from build123d import *

# Parameters (mm, degrees)
BOSS_EXTRUDE2_DEPTH   = 80
SKETCH3_W             = 20
SKETCH3_H             = 50
BOSS_EXTRUDE3_DEPTH   = 50
FILLET3_R             = 25
SKETCH8_R             = 12.5
CUT_EXTRUDE1_DEPTH    = 50
SKETCH9_R             = 7.5
CUT_EXTRUDE3_DEPTH    = 50
FILLET4_R             = 2
FILLET5_R             = 2
FILLET3_OF_MIRROR14_R = 25
FILLET4_OF_MIRROR14_R = 2
FILLET5_OF_MIRROR14_R = 2


with BuildPart() as part:
    # Sketch1 → Boss-Extrude2 (new body)
    with BuildSketch(Plane(origin=(0, 0, 0), x_dir=(0, 0, -1), z_dir=(1, 0, 0))):
        Polygon((0, 0), (-80, 0), (-80, -30), (-56.339745962, -30), (-65, -15), (-15, -15), (-23.660254038, -30), (0, -30), align=None)
    boss_extrude2 = extrude(amount=BOSS_EXTRUDE2_DEPTH)

    # Sketch3 → Boss-Extrude3 (add)
    with BuildSketch(Plane(origin=(0, 0, 0), x_dir=(1, 0, 0), z_dir=(0, 1, 0))):
        with Locations((30, -40)):
            Rectangle(SKETCH3_W, SKETCH3_H)
    boss_extrude3 = extrude(amount=BOSS_EXTRUDE3_DEPTH)

    # Fillet3
    fillet3_edges = [part.edges().sort_by_distance(p)[0] for p in [
        (30, 50, 65),
        (30, 50, 15),
    ]]
    fillet(fillet3_edges, radius=FILLET3_R - 0.0001)  # a hair under: the kernel refuses the full size

    # Sketch8 → Cut-Extrude1 (cut)
    with BuildSketch(Plane(origin=(40, 0, 0), x_dir=(0, 0, -1), z_dir=(1, 0, 0))):
        with Locations((-40, 25)):
            Circle(SKETCH8_R)
    cut_extrude1 = extrude(amount=-CUT_EXTRUDE1_DEPTH, mode=Mode.SUBTRACT)

    # Sketch9 → Cut-Extrude3 (cut)
    with BuildSketch(Plane(origin=(0, 0, 0), x_dir=(1, 0, 0), z_dir=(0, 1, 0))):
        with Locations(Location((60, -40, 0), (0, 0, 270))):
            Circle(SKETCH9_R)
    cut_extrude3 = extrude(amount=-CUT_EXTRUDE3_DEPTH, mode=Mode.SUBTRACT)

    # Fillet4
    fillet4_edges = [part.edges().sort_by_distance(p)[0] for p in [
        (30, 0, 65),
    ]]
    fillet(fillet4_edges, radius=FILLET4_R)

    # Fillet5
    fillet5_edges = [part.edges().sort_by_distance(p)[0] for p in [
        (30, 0, 15),
    ]]
    fillet(fillet5_edges, radius=FILLET5_R)

    # Mirror14: Boss-Extrude2, Boss-Extrude3, Cut-Extrude1, Cut-Extrude3 across plane
    add(boss_extrude2.mirror(Plane(origin=(0, 0, 0), x_dir=(0, 0, 1), z_dir=(1, 0, 0))))
    add(boss_extrude3.mirror(Plane(origin=(0, 0, 0), x_dir=(0, 0, 1), z_dir=(1, 0, 0))))
    add(cut_extrude1.mirror(Plane(origin=(0, 0, 0), x_dir=(0, 0, 1), z_dir=(1, 0, 0))), mode=Mode.SUBTRACT)
    add(cut_extrude3.mirror(Plane(origin=(0, 0, 0), x_dir=(0, 0, 1), z_dir=(1, 0, 0))), mode=Mode.SUBTRACT)

    # Fillet3 of Mirror14
    fillet3_of_mirror14_edges = [part.edges().sort_by_distance(p)[0] for p in [
        (-30, 50, 65),
        (-30, 50, 15),
    ]]
    fillet(fillet3_of_mirror14_edges, radius=FILLET3_OF_MIRROR14_R - 0.0001)  # a hair under: the kernel refuses the full size

    # Fillet4 of Mirror14
    fillet4_of_mirror14_edges = [part.edges().sort_by_distance(p)[0] for p in [
        (-30, 0, 65),
    ]]
    fillet(fillet4_of_mirror14_edges, radius=FILLET4_OF_MIRROR14_R)

    # Fillet5 of Mirror14
    fillet5_of_mirror14_edges = [part.edges().sort_by_distance(p)[0] for p in [
        (-30, 0, 15),
    ]]
    fillet(fillet5_of_mirror14_edges, radius=FILLET5_OF_MIRROR14_R)


solid = part.part
Could you check a few things on this model? Use its own coordinates, in mm. A direction names the side the tool comes from. Round coordinates to 2 decimals unless told otherwise and drop trailing zeros. Write each loop counter-clockwise with the first axis right and the second up, starting at its lowest first coordinate (ties: lowest second). Pieces come first, ordered by that corner, then holes. Notation, with made-up numbers: (39, -22.75) - (50, -22.75) arc R35 ccw to (50, 9.25) - close; hole circle Ø5 at (49.5, -26.75). An arc over 180 degrees is marked (long way). Use a Markdown table: item, result.
Q1. Please list where these lines run through material, in increasing order: L1, parallel to X at y = -9, z = 40; L2, parallel to Z at x = -60, y = -6; L3, parallel to X at y = 5.5, z = 19.5.
Output values:
| item | result |
|---|---|
| L1 | -80 to -67.5, -52.5 to 52.5, 67.5 to 80 |
| L2 | 0 to 32.5, 47.5 to 80 |
| L3 | -40 to -20, 20 to 40 |
Q2. For pin 1 (10 mm diameter, centred on x = 26, y = 12, fed in from -Z); pin 2 (15 mm diameter, centred on y = 25.5, z = 28, fed in from +X); pin 3 (16 mm diameter, centred on x = -33, y = 14, fed in from +Z), each with a flat end and sliding along its axis, tell me the tip position at first contact or that it passes through.
Output values:
| item | result |
|---|---|
| pin 1 | z = 15 |
| pin 2 | x = 40 |
| pin 3 | z = 65 |
Q3. For faces 1 (the flat face through (20, 13.5, 34.4)), 2 (the flat face through (30, 13, 65)), 3 (the flat face through (-40, 13.5, 34.4)), 4 (the flat face through (40, 13.5, 34.4)), which set-ups out of +Z, -Z, +X, -X, +Y, -Y let a thin tool reach every point of the face, with its end or its side?
Output values:
| item | result |
|---|---|
| face 1 | +Z, -Z, +Y |
| face 2 | +Z, +X, -X, +Y |
| face 3 | +Z, -Z, -X, +Y |
| face 4 | +Z, -Z, +X, +Y |
Q4. I want a section at B-B (y = 9.5). List the corners of the cut face in (x, z) for me.
Output values:
| item | result |
|---|---|
| outline | (-40, 15) - (-20, 15) - (-20, 65) - (-40, 65) - close; (20, 15) - (40, 15) - (40, 65) - (20, 65) - close |
Q5. I want a section at A-A (x = 64.5). List the corners of the cut face in (y, z) for me, plus the area to 3 significant figures.
Output values:
| item | result |
|---|---|
| outline | (-30, 0) - (0, 0) - (0, 34) - (-15, 34) - (-15, 15) - (-30, 23.66) - close; (-30, 56.34) - (-15, 65) - (-15, 46) - (0, 46) - (0, 80) - (-30, 80) - close |
| area | 1,600 mm2 |
Q6. I want a section at C-C (z = 44). List the corners of the cut face in (x, y) for me, plus the area to 3 significant figures.
Output values:
| item | result |
|---|---|
| outline | (-80, -15) - (-66.34, -15) - (-66.34, 0) - (-80, 0) - close; (-53.66, -15) - (53.66, -15) - (53.66, 0) - (40, 0) - (40, 13.16) - (20, 13.16) - (20, 0) - (-20, 0) - (-20, 13.16) - (-40, 13.16) - (-40, 0) - (-53.66, 0) - close; (-40, 36.84) - (-20, 36.84) - (-20, 49.68) - (-40, 49.68) - close; (20, 36.84) - (40, 36.84) - (40, 49.68) - (20, 49.68) - close; (66.34, -15) - (80, -15) - (80, 0) - (66.34, 0) - close |
| area | 3,060 mm2 |
Q7. I want a section at D-D (x = 10.5). List the corners of the cut face in (y, z) for me, plus the area to 3 significant figures.
Output values:
| item | result |
|---|---|
| outline | (-30, 0) - (0, 0) - (0, 80) - (-30, 80) - (-30, 56.34) - (-15, 65) - (-15, 15) - (-30, 23.66) - close |
| area | 1,780 mm2 |
Q8. Thinking about a two-plate mould opening in Z: for faces 5 (the flat face through (-30, 13, 15)), 6 (the cylindrical face through (-67.436, -7.395, 39.024)), 7 (the flat face through (-80, -11, 41)), which applies, released by +Z, released by -Z, zero draft, split by the parting line, or undercut?
Output values:
| item | result |
|---|---|
| face 5 | released by -Z |
| face 6 | undercut |
| face 7 | zero draft |
